Design review of the part built by this model. Coordinates are the model's own, in mm. Face numbers are marked on the shaded views. Give positions to 0.01 mm unless a question says otherwise; leave off trailing zeros. Write each loop counter-clockwise with the first axis right and the second up, starting at its lowest first coordinate (ties: lowest second). Pieces come first, ordered by that corner, then holes. Notation, with made-up numbers: (-5.5, -10) - (30.5, -10) arc R15 ccw to (30.5, 3) - close; hole circle Ø3 at (67, 82). An arc over 180 degrees is marked (long way). Use a Markdown table: item, result. Add a question column.
```python
from build123d import *

# Parameters (mm, degrees)
F0_R     = 52.3875
F1_DEPTH = 3.175
F2_R     = 46.99
F3_DEPTH = 177.8
F5_R     = 43.815
F6_DEPTH = 177.8


with BuildPart() as f1:
    # F0 (on Top) → F1 (new body)
    with BuildSketch(Plane.XY):
        Circle(F0_R)
    extrude(amount=F1_DEPTH)

    # F2 (on Top) → F3 (join)
    with BuildSketch(Plane.XY):
        Circle(F2_R)
    extrude(amount=-F3_DEPTH)

    # F5 (on offset) → F6 (cut)
    with BuildSketch(Plane.XY.offset(3.175)):
        Circle(F5_R)
    extrude(amount=-F6_DEPTH, mode=Mode.SUBTRACT)


solid = f1.part
```
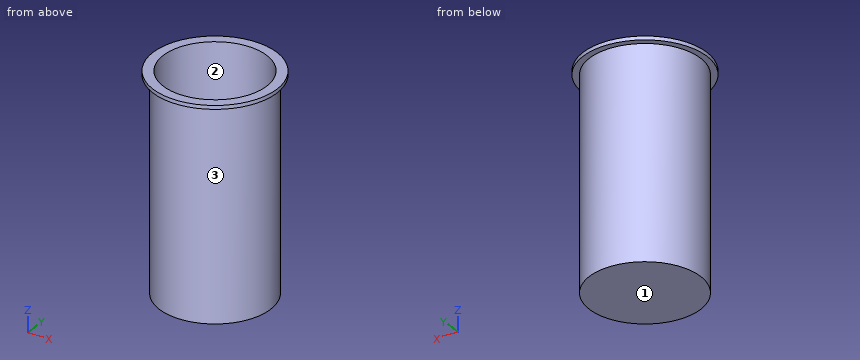
(1) Add section C-C (z = -43). State the section outline as (x, y) points (3 decimals), and give its area (3 significant figures).
(2) Mouldability with a two-part tool opening along Y and no side actions: class the marked faces 1, 2 and 3 as +Y half, -Y half, draft (parallel to the pull), parting line (faces both ways), or undercut.
(3) Insertion check: pin 1 (3 mm diameter, centred on x = -24.5, z = -26, fed in from +Y); pin 2 (2 mm diameter, centred on y = -28.5, z = -27.5, fed in from -X); pin 3 (1.5 mm diameter, centred on x = -28.5, z = -79, fed in from -Y). Each pin has a flat end and moves straight along its axis. Give the tip position at first contact, or say it passes through.
(4) Add section A-A (x = 0). State the section outline as (y, z) points (1 decimal), and give its area (3 significant figures).
(5) For line 1 along X through (y, z) = (1.5, -158.5); line 2 along Y through (x, z) = (-2, -76.5); line 3 along Z through (x, y) = (-18, 45.5) (3 decimals), list the stretches that pass through material, from the lowest coordinate up.
Answers follow:
| question | item | result |
|---|---|---|
| 1 | outline | circle Ø93.98 at (0, 0); hole circle Ø87.63 at (0, 0) |
| 1 | area | 906 mm^2 |
| 2 | face 1 | draft |
| 2 | face 2 | undercut |
| 2 | face 3 | parting line |
| 3 | pin 1 | y = 40.98 |
| 3 | pin 2 | x = -38.1 |
| 3 | pin 3 | y = -37.92 |
| 4 | outline | (-52.4, 0) - (-47, 0) - (-47, -177.8) - (47, -177.8) - (47, 0) - (52.4, 0) - (52.4, 3.2) - (43.8, 3.2) - (43.8, -174.6) - (-43.8, -174.6) - (-43.8, 3.2) - (-52.4, 3.2) - close |
| 4 | area | 1,460 mm^2 |
| 5 | line 1 | -46.97 to -43.79, 43.79 to 46.97 |
| 5 | line 2 | -46.95 to -43.77, 43.77 to 46.95 |
| 5 | line 3 | 0 to 3.175 |
